Part model, mm, in its own coordinate system. Face numbers are marked on the shaded views. A direction names the side the tool comes from. Coordinates: 2 decimals unless noted, no trailing zeros. Loops run counter-clockwise (first coordinate to the right, second up) from the corner with the lowest first, then second, coordinate; pieces in that order, holes last. Notation, with made-up numbers: M 45,82 L 76,82 A27 cw 76,100 Z; hole C 82,32.5 d9. An arc over 180 degrees is marked long. Answer as a JSON object with one key per item and string values. Group by question number.
1. Saw through at B-B on y = 18.5. Write the cut outline in (x, z), then the cut area to 3 significant figures.
2. Saw through at D-D on z = -9. Write the cut outline in (x, y).
3. Drill centre lines: L1, parallel to Y at x = 27, z = 5; L2, parallel to X at y = 20.5, z = 10.5; L3, parallel to Y at x = 13, z = -11. Where is each one in solid material? Low to high.
4. Saw through at A-A on z = 3.5. Write the cut outline in (x, y).
5. Mould opens along Y. For the marked faces 1, 2, 3 and 4 say: released by +Y, released by -Y, zero draft, split by the parting line, or undercut.
6. Saw through at C-C on x = 21. Write the cut outline in (y, z), then the cut area to 3 significant figures.
7. Drop flat-ended pins along their axis: pin 1 Ø3 at (x, z) = (8, -6) entering from +Y; pin 2 Ø14.5 at (x, z) = (19, -6) entering from -Y; pin 3 Ø5.5 at (y, z) = (33, -1.5) entering from -X; pin 4 Ø4 at (x, z) = (17.5, 14) entering from +Y. Give the stop position or say it passes through.
8. 3-axis set-ups, long thin cutter, end or side, ignore diameter. For the marked faces 5, 6 and 7: which of +Z, -Z, +X, -X, +Y, -Y reach the whole face in a straight line?
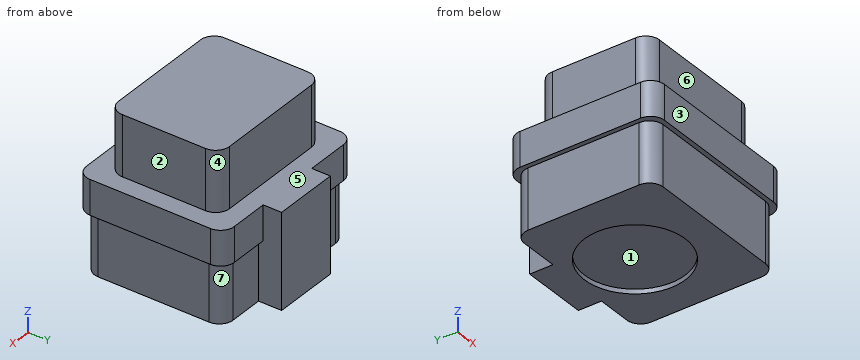
from build123d import *

# Parameters (mm, degrees)
SKETCH_1_W          = 38
SKETCH_1_H          = 32
EXTRUDE_1_DEPTH     = 7.5
SKETCH_2_W          = 30
SKETCH_2_H          = 24
EXTRUDE_2_DEPTH     = 13
SKETCH_3_W          = 36
SKETCH_3_H          = 30
EXTRUDE_3_DEPTH     = 13
FILLET_1_R          = 3
SKETCH_4_W          = 14.251967781
SKETCH_4_H          = 20.5
EXTRUDE_4_DEPTH     = 5
SKETCH_5_R          = 10.910611056
CUT_EXTRUDE_1_DEPTH = 1


with BuildPart() as part:
    # ｽｹｯﾁ1 → ﾎﾞｽ - 押し出し1 (new body)
    with BuildSketch(Plane.XY):
        with Locations((19, 16)):
            Rectangle(SKETCH_1_W, SKETCH_1_H)
    extrude(amount=EXTRUDE_1_DEPTH)

    # ｽｹｯﾁ2 → ﾎﾞｽ - 押し出し2 (add)
    with BuildSketch(Plane.XY.offset(7.5)):
        with Locations((19, 16)):
            Rectangle(SKETCH_2_W, SKETCH_2_H)
    extrude(amount=EXTRUDE_2_DEPTH)

    # ｽｹｯﾁ3 → ﾎﾞｽ - 押し出し3 (add)
    with BuildSketch(Plane(origin=(0, 0, 0), x_dir=(-1, 0, 0), z_dir=(0, 0, -1))):
        with Locations((-19, 16)):
            Rectangle(SKETCH_3_W, SKETCH_3_H)
    extrude(amount=EXTRUDE_3_DEPTH)

    # ﾌｨﾚｯﾄ1
    fillet_1_edges = [part.edges().sort_by_distance(p)[0] for p in [
        (34, 28, 14),
        (4, 28, 14),
        (4, 4, 14),
        (34, 4, 14),
        (37, 1, -6.5),
        (1, 1, -6.5),
        (1, 31, -6.5),
        (37, 31, -6.5),
        (0, 32, 3.75),
        (38, 32, 3.75),
        (38, 0, 3.75),
        (0, 0, 3.75),
    ]]
    fillet(fillet_1_edges, radius=FILLET_1_R)

    # ｽｹｯﾁ4 → ﾎﾞｽ - 押し出し4 (add)
    with BuildSketch(Plane(origin=(0, 31, 0), x_dir=(1, 0, 0), z_dir=(0, 1, 0))):
        with Locations((19.433755542, 2.75)):
            Rectangle(SKETCH_4_W, SKETCH_4_H)
    extrude(amount=EXTRUDE_4_DEPTH)

    # ｽｹｯﾁ5 → ｶｯﾄ - 押し出し1 (cut)
    with BuildSketch(Plane(origin=(0, 0, -13), x_dir=(-1, 0, 0), z_dir=(0, 0, -1))):
        with Locations((-19.433755541, 18.5)):
            Circle(SKETCH_5_R)
    extrude(amount=-CUT_EXTRUDE_1_DEPTH, mode=Mode.SUBTRACT)


solid = part.part
Outcome:
{
 "1": {"outline": "M 0,0 L 1,0 L 1,-13 L 8.52,-13 L 8.52,-12 L 30.34,-12 L 30.34,-13 L 37,-13 L 37,0 L 38,0 L 38,7.5 L 34,7.5 L 34,20.5 L 4,20.5 L 4,7.5 L 0,7.5 Z", "area": "1,120 mm²"},
 "2": {"outline": "M 1,4 A3 ccw 4,1 L 34,1 A3 ccw 37,4 L 37,28 A3 ccw 34,31 L 26.56,31 L 26.56,36 L 12.31,36 L 12.31,31 L 4,31 A3 ccw 1,28 Z"},
 "3": {"L1": "y = 0 to 32", "L2": "x = 4 to 34", "L3": "y = 1 to 36"},
 "4": {"outline": "M 0,3 A3 ccw 3,0 L 35,0 A3 ccw 38,3 L 38,29 A3 ccw 35,32 L 26.56,32 L 26.56,36 L 12.31,36 L 12.31,32 L 3,32 A3 ccw 0,29 Z"},
 "5": {"face 1": "undercut", "face 2": "zero draft", "face 3": "released by -Y", "face 4": "released by +Y"},
 "6": {"outline": "M 0,0 L 1,0 L 1,-13 L 7.7,-13 L 7.7,-12 L 29.3,-12 L 29.3,-13 L 36,-13 L 36,7.5 L 28,7.5 L 28,20.5 L 4,20.5 L 4,7.5 L 0,7.5 Z", "area": "1,020 mm²"},
 "7": {"pin 1": "stops at y = 31", "pin 2": "stops at y = 0", "pin 3": "stops at x = 0.52", "pin 4": "stops at y = 28"},
 "8": {"face 5": "+Z", "face 6": "+Z, +X, -X, -Y", "face 7": "-Z, +X, +Y"}
}
